```python
from build123d import *

# Parameters (mm, degrees)
SKETCH1_R          = 85
WHEEL_DEPTH        = 60
FILLET1_R          = 25
SKETCH4_R          = 10
CUT_EXTRUDE1_DEPTH = 135.350288489


with BuildPart() as part:
    # Sketch1 → WHEEL (new body)
    with BuildSketch(Plane.XY):
        Circle(SKETCH1_R)
    extrude(amount=WHEEL_DEPTH)

    # Fillet1
    fillet1_edges = [part.edges().sort_by_distance(p)[0] for p in [
        (-85, 0, 0),
        (-85, 0, 60),
    ]]
    fillet(fillet1_edges, radius=FILLET1_R)

    # Sketch4 → Cut-Extrude1 (cut, through all)
    with BuildSketch(Plane(origin=(0, 0, 0), x_dir=(-1, 0, 0), z_dir=(0, 0, -1))):
        Circle(SKETCH4_R)
    extrude(amount=-CUT_EXTRUDE1_DEPTH, mode=Mode.SUBTRACT)


solid = part.part
```
Geometry check sheet. Reference: the model listing, model coordinates, mm. Round coordinates to 2 decimals unless told otherwise and drop trailing zeros. Order: outer loops, then holes, each group sorted by start corner. A loop starts at its lowest first (then second) coordinate and runs counter-clockwise, first axis right, second up. Notation, with made-up numbers: (1, 80) - (40, 80) arc R22 ccw to (40, 90) - close; hole circle Ø10 at (52.5, 45). An arc over 180 degrees is marked (long way). Use a Markdown table: item, result. Add a question column.
(1) Depth check by flat-ended pin: pin 1 (2 mm diameter, centred on y = 62.5, z = 29.5, fed in from -X); pin 2 (12 mm diameter, centred on x = -50, z = 31, fed in from -Y); pin 3 (10 mm diameter, centred on x = 20, z = 52.5, fed in from -Y). Enter the tip coordinate at first touch or a pass-through.
(2) Release check for a two-part mould opening along Y. For faces 1 (the cylindrical face through (2.17, -9.76, 29.58)), 2 (the flat face through (12, 1, 60)), 3 (the cylindrical face through (-67.453, -51.721, 29.93)) record: pulls with the +Y half, pulls with the -Y half, needs draft (parallel to the pull), parting line crosses it, or undercut.
(3) Sectioned sample at C-C, the plane z = 47. Enter the section's corners in (x, y), and give its area (3 significant figures).
(4) Material ranges on line 1 along Y through (x, z) = (0, 12); line 2 along Y through (x, z) = (0, 46); line 3 along X through (y, z) = (-3, 17), recorded low to high. Write a range as [from, to].
(5) Sectioned sample at D-D, the plane z = 7. Enter the section's corners in (x, y).
(6) Sectioned sample at A-A, the plane x = 0. Enter the section's corners in (y, z), and give its area (3 significant figures).
Answers below:
| question | item | result |
|---|---|---|
| 1 | pin 1 | x = -58.67 |
| 1 | pin 2 | y = -72.73 |
| 1 | pin 3 | y = -79.39 |
| 2 | face 1 | undercut |
| 2 | face 2 | needs draft |
| 2 | face 3 | parting line crosses it |
| 3 | outline | circle Ø163.86 at (0, 0); hole circle Ø20 at (0, 0) |
| 3 | area | 20,800 mm² |
| 4 | line 1 | [-81.35, -10], [10, 81.35] |
| 4 | line 2 | [-82.45, -10], [10, 82.45] |
| 4 | line 3 | [-83.63, -9.54], [9.54, 83.63] |
| 5 | outline | circle Ø154.7 at (0, 0); hole circle Ø20 at (0, 0) |
| 6 | outline | (-85, 25) arc R25 ccw to (-60, 0) - (-10, 0) - (-10, 60) - (-60, 60) arc R25 ccw to (-85, 35) - close; (10, 0) - (60, 0) arc R25 ccw to (85, 25) - (85, 35) arc R25 ccw to (60, 60) - (10, 60) - close |
| 6 | area | 8,460 mm² |
